Verification items for the finished model (mm, model axes). Face numbers are marked on the shaded views. A direction names the side the tool comes from. Round coordinates to 2 decimals unless told otherwise and drop trailing zeros. Order: outer loops, then holes, each group sorted by start corner. A loop starts at its lowest first (then second) coordinate and runs counter-clockwise, first axis right, second up. Notation, with made-up numbers: (84, 80.5) -> (138, 80.5) arc R7 ccw to (138, 86.5) -> close; hole circle Ø6 at (24.5, 80). An arc over 180 degrees is marked (long way). Answer in a Markdown table with one row per item. Add a question column.
```python
from build123d import *

# Parameters (mm, degrees)
F0_W        = 60.96
F0_H        = 4.064
F1_DEPTH    = 60.96
F3_DEPTH    = 25.4
F6_DEPTH    = 60.96
F7_T4_DEPTH = 53.34
F7_S5_R     = 30.988
F7_T6_DEPTH = 44
F7_S7_R     = 30.48
F7_T8_DEPTH = 44
F8_W        = 60.96
F8_H        = 4.064
F9_DEPTH    = 6.35
F10_W       = 3.175
F10_H       = 60.96
F11_DEPTH   = 10
F4_R        = 2.0955
F14_DEPTH   = 65.025
F13_R       = 2.5
F15_DEPTH   = 25.4
F12_R       = 2.5
F16_DEPTH   = 25.4


# Not quite as in the source:
# - a fillet or chamfer that OpenCascade refuses, or shapes differently, is made with other operations: its cross-section is extruded or revolved along the edge and cut away or added


with BuildPart() as f1:
    # F0 (on Right) → F1 (new body)
    with BuildSketch(Plane.YZ):
        with Locations((2.5902520865, 22.5415869818)):
            Rectangle(F0_W, F0_H)
    extrude(amount=F1_DEPTH)

    # F2 (on face) → F3 (cut)
    with BuildSketch(Plane.XY.offset(24.5735869818)):
        with BuildLine():
            Line((16.002, -24.0797479135), (44.958, -24.0797479135))
            ThreePointArc((44.958, -24.0797479135), (51.934072902, -18.8638208155), (57.15, -11.8877479135))
            Line((57.15, -11.8877479135), (57.15, 17.0682520865))
            ThreePointArc((57.15, 17.0682520865), (51.934072902, 24.0443249885), (44.958, 29.2602520865))
            Line((44.958, 29.2602520865), (16.002, 29.2602520865))
            ThreePointArc((16.002, 29.2602520865), (9.0409528702, 24.0292992163), (3.81, 17.0682520865))
            Line((3.81, 17.0682520865), (3.81, -11.8877479135))
            ThreePointArc((3.81, -11.8877479135), (9.025927098, -18.8638208155), (16.002, -24.0797479135))
        make_face()
    extrude(amount=-F3_DEPTH, mode=Mode.SUBTRACT)

    # F5 (on face) → F6 (join)
    with BuildSketch(Plane.XZ.offset(27.8897479135)):
        Polygon((30.48, -40.4504130182), (30.48, 20.5095869818), (0, 20.5095869818), align=None)
    extrude(amount=-F6_DEPTH)

    # F7: chamfer of 60.96 x 26.67 on 1 edges, made by hand


with BuildPart() as f7_tool2:
    # F7_s3 → F7_t4 (new body)
    with BuildSketch(Plane.XZ.offset(24.0797479135)):
        Polygon((3.81, 20.5095869818), (30.48, -40.4504130182), (30.48, 20.5095869818), align=None)
    extrude(amount=-F7_T4_DEPTH)

    # F7_s5 → F7_t6 (intersect, symmetric)
    with BuildSketch(Plane.XY.offset(-10)):
        with Locations((30.9527778056, 2.1174742809)):
            Circle(F7_S5_R)
    extrude(amount=F7_T6_DEPTH, both=True, mode=Mode.INTERSECT)

    # F7_s7 → F7_t8 (intersect, symmetric)
    with BuildSketch(Plane.XY.offset(-10)):
        with Locations((30.5785417886, 2.6887938751)):
            Circle(F7_S7_R)
    extrude(amount=F7_T8_DEPTH, both=True, mode=Mode.INTERSECT)


with BuildPart() as f1_1:
    add(f1.part)

    # F7_t1: cut F7_tool2
    add(f7_tool2.part, mode=Mode.SUBTRACT)

    # F8 (on face) → F9 (join)
    with BuildSketch(Plane.YZ.offset(60.96)):
        with Locations((2.5902520865, 22.5415869818)):
            Rectangle(F8_W, F8_H)
    extrude(amount=F9_DEPTH)

    # F10 (on face) → F11 (join)
    with BuildSketch(Plane(origin=(0, 0, 20.5095869818), x_dir=(1, 0, 0), z_dir=(0, 0, -1))):
        with Locations((65.7225, -2.5902520865)):
            Rectangle(F10_W, F10_H)
    extrude(amount=F11_DEPTH)

    # F4 (on face) → F14 (cut, through all)
    with BuildSketch(Plane.XY.offset(24.5735869818)):
        with Locations((55.372, -22.3017479135)):
            Circle(F4_R)
        with Locations((55.372, 27.4822520865)):
            Circle(F4_R)
        with Locations((5.588, -22.3017479135)):
            Circle(F4_R)
        with Locations((5.588, 27.4822520865)):
            Circle(F4_R)
    extrude(amount=-F14_DEPTH, mode=Mode.SUBTRACT)

    # F13 (on face) → F15 (cut)
    with BuildSketch(Plane(origin=(64.135, 0, 0), x_dir=(0, -1, 0), z_dir=(-1, 0, 0))):
        with Locations((23.3897479135, 16.1365869818)):
            Circle(F13_R)
    extrude(amount=-F15_DEPTH, mode=Mode.SUBTRACT)

    # F12 (on face) → F16 (cut)
    with BuildSketch(Plane(origin=(64.135, 0, 0), x_dir=(0, -1, 0), z_dir=(-1, 0, 0))):
        with Locations((-28.5702520865, 16.1365869818)):
            Circle(F12_R)
    extrude(amount=-F16_DEPTH, mode=Mode.SUBTRACT)


solid = f1_1.part
```
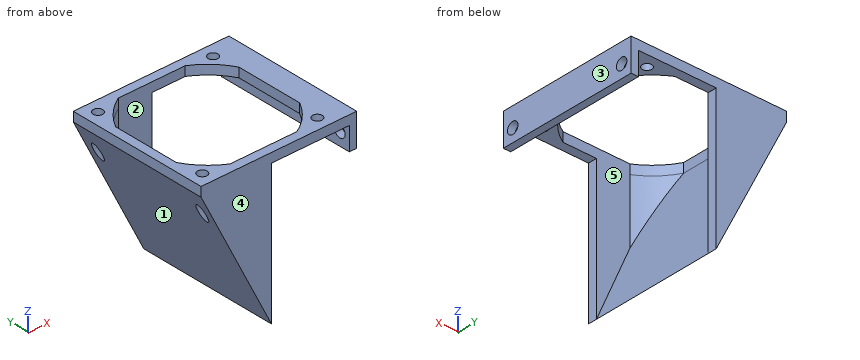
1) Depth check by flat-ended pin: P1, Ø23, axis at x = 37.5, z = -24, coming from the -Y side; P2, Ø1.1, axis at y = 31, z = -16, coming from the +X side; P3, Ø4, axis at y = 28.57, z = 16.14, coming from the -X side; P4, Ø3, axis at x = 33, z = -6.5, coming from the -Y side. Enter the tip coordinate at first touch or a pass-through.
2) Cross-section at D-D, the plane x = 15. Record the boundary of the cut face in (y, z).
3) Draft check along Y on the marked faces 3, 4 and 5. Enter one of: +Y half, -Y half, draft (parallel to the pull), parting line (faces both ways), or undercut.
4) Cross-section at C-C, the plane z = 9. Record the boundary of the cut face in (x, y), and give its area (3 significant figures).
5) Thickness scan on L1, parallel to Y at x = 16.5, z = 1; L2, parallel to X at y = 9, z = 22.5; L3, parallel to Y at x = 6.5, z = 16.5. Record the ranges inside material, lowest first. Write a range as [from, to].
6) Cross-section at A-A, the plane y = 5. Record the boundary of the cut face in (x, z) (3 decimals), and give its area (3 significant figures).
7) Cross-section at B-B, the plane x = 46. Record the boundary of the cut face in (y, z).
8) Tool access check on the marked faces 1 and 2. Record the directions out of +Z, -Z, +X, -X, +Y, -Y that give a thin tool (end or side, any length) a straight path to the whole face; none if there is none.
Results below:
| question | item | result |
|---|---|---|
| 1 | P1 | y = -27.89 |
| 1 | P2 | x = 30.48 |
| 1 | P3 | x = 1.18 |
| 1 | P4 | through |
| 2 | outline | (-27.89, -9.49) -> (33.07, -9.49) -> (33.07, 24.57) -> (28.68, 24.57) -> (28.68, -5.07) -> (-23.51, -5.07) -> (-23.51, 24.57) -> (-27.89, 24.57) -> close |
| 3 | face 3 | draft |
| 3 | face 4 | -Y half |
| 3 | face 5 | undercut |
| 4 | outline | (5.75, -27.89) -> (30.48, -27.89) -> (30.48, -24.08) -> (16, -24.08) arc R30.48 cw to (8.85, -18.68) -> (8.85, 23.83) arc R30.99 cw to (16, 29.26) -> (30.48, 29.26) -> (30.48, 33.07) -> (5.75, 33.07) -> (5.75, 29.57) arc R2.1 cw to (5.75, 25.39) -> (5.75, -20.21) arc R2.1 cw to (5.75, -24.39) -> close |
| 4 | area | 376 mm² |
| 5 | L1 | [-27.89, -24.08], [29.26, 33.07] |
| 5 | L2 | [0, 3.81], [57.15, 67.31] |
| 5 | L3 | [-27.89, -24.19], [-20.42, -16], [21.15, 25.6], [29.37, 33.07] |
| 6 | outline | (0, 20.51) -> (30.48, -40.45) -> (3.81, 20.51) -> (3.81, 24.574) -> (0, 24.574) -> close; (57.15, 20.51) -> (64.135, 20.51) -> (64.135, 10.51) -> (67.31, 10.51) -> (67.31, 24.574) -> (57.15, 24.574) -> close |
| 6 | area | 205 mm² |
| 7 | outline | (-27.89, 20.51) -> (-23.49, 20.51) -> (-23.49, 24.57) -> (-27.89, 24.57) -> close; (28.67, 20.51) -> (33.07, 20.51) -> (33.07, 24.57) -> (28.67, 24.57) -> close |
| 8 | face 1 | -Z, -X, +Y, -Y |
| 8 | face 2 | +Z |
